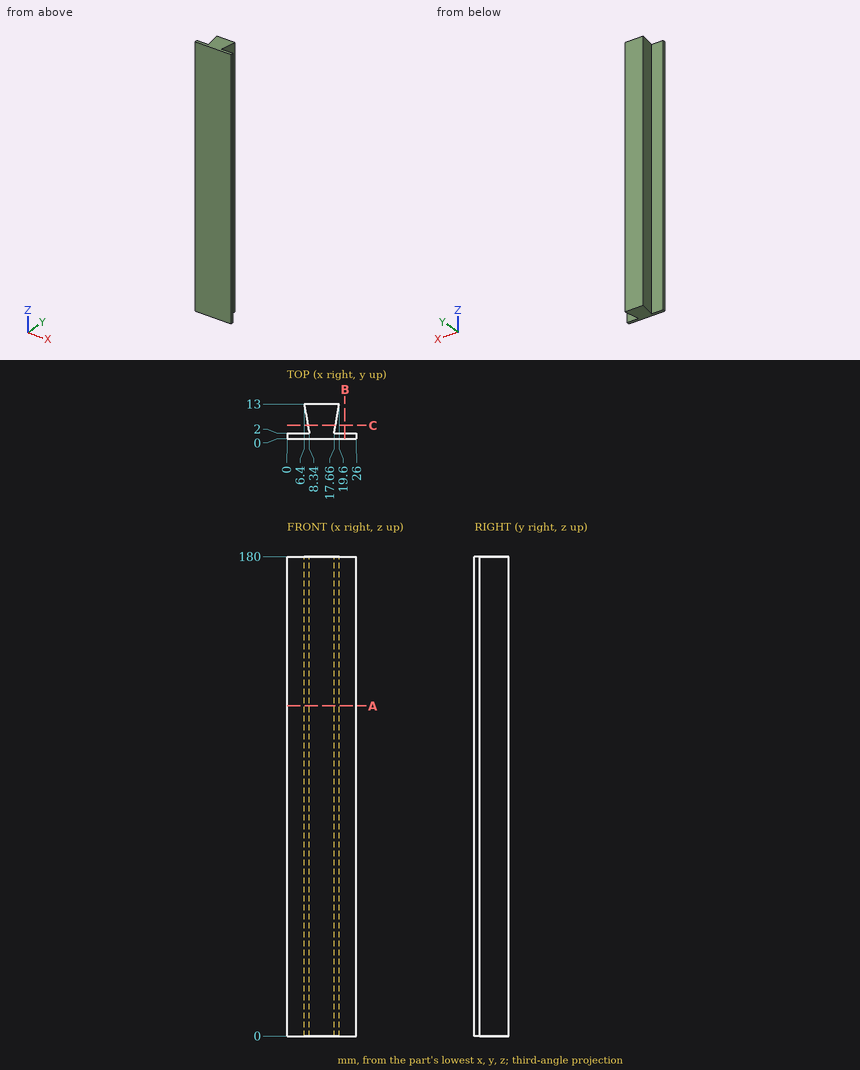
The drawing under review shows one solid part. Ordinate dimensions are in mm from its lowest x, y, z. Coordinates: 2 decimals unless noted, no trailing zeros. Order: outer loops, then holes, each group sorted by start corner. A loop starts at its lowest first (then second) coordinate and runs counter-clockwise, first axis right, second up. Notation, with made-up numbers: (-40, -14) -> (-22, -14) arc R30 ccw to (-22, 21) -> close; hole circle Ø2 at (52.25, 65). An arc over 180 degrees is marked (long way). Use CSV: the item, a comma, the result in double quotes. Start each with the question number.
Item 1: Wall thickness on probe 1 along Y at (x, z) = (5.75, 87); probe 2 along X at (y, z) = (3.5, 63.5) (1 decimal); probe 3 along X at (y, z) = (4.75, 135) (1 decimal): over which ranges is each line inside the solid? List them lowest first.
Item 2: We need section B-B, the plane x = 21.75. Give the boundary of the cut face in (y, z), then the cut area to 3 significant figures.
Item 3: Insertion check: pin 1 (1.5 mm diameter, centred on x = 20.5, z = 84.5, fed in from -Y); pin 2 (4 mm diameter, centred on y = 10, z = 118, fed in from -X); pin 3 (3 mm diameter, centred on y = 7, z = 69, fed in from +X). Each pin has a flat end and moves straight along its axis. Give the tip position at first contact, or say it passes through.
Item 4: We need section A-A, the plane z = 124. Give the boundary of the cut face in (x, y).
Item 5: We need section C-C, the plane y = 5. Give the boundary of the cut face in (x, z), then the cut area to 3 significant figures.
Derived:
1,probe 1,"y = 0 to 2"
1,probe 2,"x = 8.1 to 17.9"
1,probe 3,"x = 7.9 to 18.1"
2,outline,"(0, 0) -> (2, 0) -> (2, 180) -> (0, 180) -> close"
2,area,"360 mm^2"
3,pin 1,"stops at y = 0"
3,pin 2,"stops at x = 6.58"
3,pin 3,"stops at x = 18.81"
4,outline,"(0, 0) -> (26, 0) -> (26, 2) -> (17.66, 2) -> (19.6, 13) -> (6.4, 13) -> (8.34, 2) -> (0, 2) -> close"
5,outline,"(7.81, 0) -> (18.19, 0) -> (18.19, 180) -> (7.81, 180) -> close"
5,area,"1,870 mm^2"
